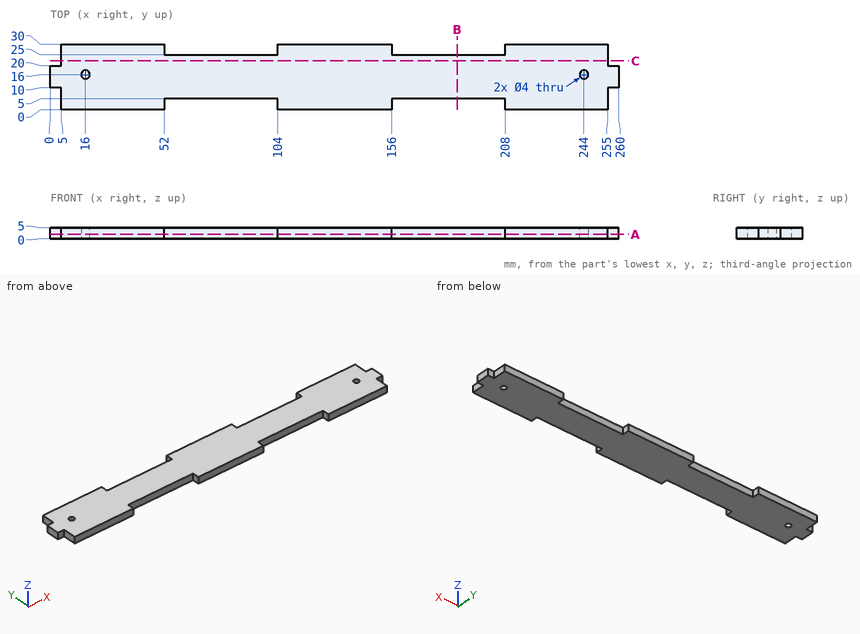
Job drawing, mm, ordinate dimensions from the low corner. One solid piece. Give positions to 0.01 mm unless a question says otherwise; leave off trailing zeros. Order: outer loops, then holes, each group sorted by start corner. A loop starts at its lowest first (then second) coordinate and runs counter-clockwise, first axis right, second up. Notation, with made-up numbers: (4, 58.25) -> (59, 58.25) arc R17 ccw to (59, 69.25) -> close; hole circle Ø7 at (60, 23). An arc over 180 degrees is marked (long way). Return JSON: item names as keys, results as strings.
Q1. Saw through at A-A (z = 1.9). Count the separate pieces of the cut face and the enclosed holes in it, then the cut area to 3 significant figures.
Working result:
{"separate pieces": "1", "enclosed holes": "2", "area": "6,530 mm²"}
Q2. Drill centre lines: line 1 (X direction, y = 16.25, z = 3.6); line 2 (Y direction, x = 16, z = 1.7); line 3 (X direction, y = 24.5, z = 3.05). Where is each one in solid material? Low to high.
Working result:
{"line 1": "0 to 14.02, 17.98 to 242.02, 245.98 to 260", "line 2": "0 to 14, 18 to 30", "line 3": "5 to 255"}
Q3. Saw through at B-B (x = 186). Write the cut outline in (y, z), then the cut area to 3 significant figures.
Working result:
{"outline": "(5, 0) -> (25, 0) -> (25, 5) -> (5, 5) -> close", "area": "100 mm²"}
Q4. Flat gauge pins, fed straight in: pin 1 (3 mm diameter, centred on y = 7.5, z = 1.5, fed in from -X); pin 2 (1.5 mm diameter, centred on x = 1.5, z = 2.5, fed in from +Y); pin 3 (2.5 mm diameter, centred on x = 258.5, z = 2, fed in from -Y); pin 4 (3 mm diameter, centred on x = 16, y = 16, fed in from +Z). Where does each tip first touch, or does it go through?
Working result:
{"pin 1": "x = 5", "pin 2": "y = 20", "pin 3": "y = 10", "pin 4": "through"}
Q5. Saw through at C-C (y = 22.25). Write the cut outline in (x, z).
Working result:
{"outline": "(5, 0) -> (255, 0) -> (255, 5) -> (5, 5) -> close"}
